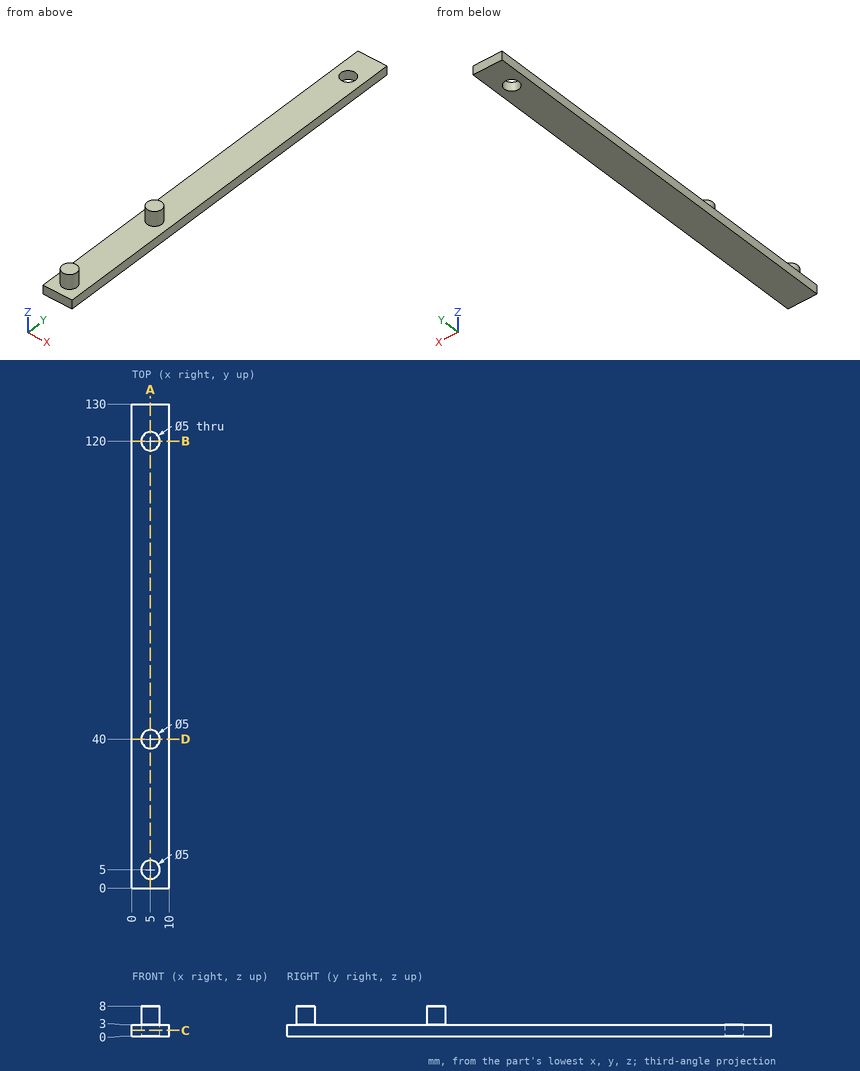
For this review, use the dimensioned drawing (mm, ordinates from the lowest corner) and the shaded views. Give positions to 0.01 mm unless a question says otherwise; leave off trailing zeros. Loops run counter-clockwise (first coordinate to the right, second up) from the corner with the lowest first, then second, coordinate; pieces in that order, holes last. Notation, with made-up numbers: (-34.5, -10.75) - (-11.5, -10.75) arc R23 ccw to (-11.5, -0.75) - close; hole circle Ø2 at (24, 50.25). An arc over 180 degrees is marked (long way). Write each question's results on one line, items separated by ' | '.
(1) Take a section at D-D (y = 40). Give the boundary of the cut face in (x, z).
Conclusion:
outline: (0, 0) - (10, 0) - (10, 3) - (7.5, 3) - (7.5, 8) - (2.5, 8) - (2.5, 3) - (0, 3) - close
(2) For line 1 along Y through (x, z) = (5, 1.35); line 2 along Z through (x, y) = (3.25, 103.5); line 3 along Y through (x, z) = (4, 7.5), list the stretches that pass through material, from the lowest coordinate up.
Conclusion:
line 1: 0 to 117.5, 122.5 to 130 | line 2: 0 to 3 | line 3: 2.71 to 7.29, 37.71 to 42.29
(3) For pin 1 Ø4 at (x, y) = (3, 112.5) entering from -Z; pin 2 Ø5 at (x, y) = (7.5, 63) entering from +Z; pin 3 Ø2 at (y, z) = (93, 5.5) entering from +X, all flat-tipped, find the tip position at first contact; note any pin that passes through.
Conclusion:
pin 1: z = 0 | pin 2: z = 3 | pin 3: through
(4) Take a section at C-C (z = 1.5). Give the boundary of the cut face in (x, y).
Conclusion:
outline: (0, 0) - (10, 0) - (10, 130) - (0, 130) - close; hole circle Ø5 at (5, 120)
(5) Take a section at B-B (y = 120). Give the boundary of the cut face in (x, z).
Conclusion:
outline: (0, 0) - (2.5, 0) - (2.5, 3) - (0, 3) - close; (7.5, 0) - (10, 0) - (10, 3) - (7.5, 3) - close
(6) Take a section at A-A (x = 5). Give the boundary of the cut face in (y, z).
Conclusion:
outline: (0, 0) - (117.5, 0) - (117.5, 3) - (42.5, 3) - (42.5, 8) - (37.5, 8) - (37.5, 3) - (7.5, 3) - (7.5, 8) - (2.5, 8) - (2.5, 3) - (0, 3) - close; (122.5, 0) - (130, 0) - (130, 3) - (122.5, 3) - close
